Design review of the part built by this model. Coordinates are the model's own, in mm. Coordinates: 2 decimals unless noted, no trailing zeros. Loops run counter-clockwise (first coordinate to the right, second up) from the corner with the lowest first, then second, coordinate; pieces in that order, holes last. Notation, with made-up numbers: M -26,63 L -6,63 A20 ccw -6,87 Z; hole C 56.25,3 d10. An arc over 180 degrees is marked long. Write item = value, one per line. Start each with the question number.
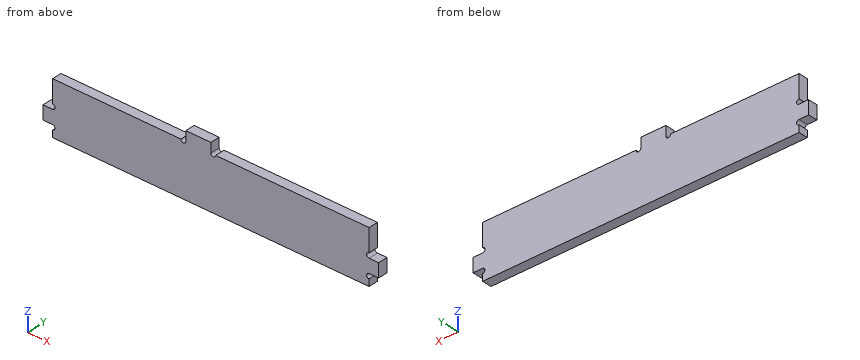
Autodesk Inventor part; units mm, degrees
ref_plane "YZ Plane" through (0, 0, 0) normal (1, 0, 0) x (0, 1, 0)
ref_plane "XZ Plane" through (0, 0, 0) normal (0, 1, 0) x (-1, 0, 0)
ref_plane "XY Plane" through (0, 0, 0) normal (0, 0, 1) x (1, 0, 0)
sketch "Sketch1" plane through (0, 0, 0) normal (0, 1, 0) x (-1, 0, 0)
  arc A0 (54.4292, -38.5976) -> (54.4292, -42.0976) centre (54.4292, -40.3476) ccw
  arc A1 (54.4292, -25.0976) -> (54.4292, -28.5976) centre (54.4292, -26.8476) ccw
  line L0 (61.4292, -38.5976) -> (61.4292, -28.5976)
  line L1 (-42.6541, -8.5976) -> (-42.6541, -1.5976)
  line L2 (61.4292, -28.5976) -> (54.4292, -28.5976)
  line L3 (61.4292, -38.5976) -> (54.4292, -38.5976)
  line L4 (54.4292, -25.0976) -> (54.4292, -8.5976)
  line L5 (54.4292, -42.0976) -> (54.4292, -47.0976)
  line L6 (-60.9041, -44.0976) -> (-60.9041, -33.5976)
  arc A2 (-176.2375, -42.0976) -> (-176.2375, -38.5976) centre (-176.2375, -40.3476) ccw
  arc A3 (-176.2375, -28.5976) -> (-176.2375, -25.0976) centre (-176.2375, -26.8476) ccw
  line L7 (-183.2375, -38.5976) -> (-183.2375, -28.5976)
  line L8 (-183.2375, -28.5976) -> (-176.2375, -28.5976)
  line L9 (-183.2375, -38.5976) -> (-176.2375, -38.5976)
  line L10 (-176.2375, -25.0976) -> (-176.2375, -8.5976)
  line L11 (-176.2375, -42.0976) -> (-176.2375, -47.0976)
  line L12 (54.4292, -47.0976) -> (-176.2375, -47.0976)
  arc A4 (-42.6541, -8.5976) -> (-39.1541, -8.5976) centre (-40.9041, -8.5976) ccw
  line L13 (-39.1541, -8.5976) -> (54.4292, -8.5976)
  line L14 (-60.9041, -1.5976) -> (-60.9041, -8.5976)
  arc A5 (-64.4041, -8.5976) -> (-60.9041, -8.5976) centre (-62.6541, -8.5976) ccw
  line L15 (-64.4041, -8.5976) -> (-176.2375, -8.5976)
  line L16 (-42.6541, -1.5976) -> (-60.9041, -1.5976)
  point P0 (0, 0)
  dimension "d2" = 3.5
  dimension "d5" = 3.5
  dimension "d9" = 7
  dimension "d11" = 10
  dimension "d32" = 5
  dimension "d33" = 230.6667
  dimension "d36" = 7
  dimension "d42" = 3.5
  dimension "d43" = 97.0833
  dimension "d44" = 3.5
  dimension "d45" = 18.25
  dimension "d46" = 20
extrude "Extrusion1" add sketch "Sketch1" along normal blind 7
properties part number "Level 1 Support Mid" material "Wood (Maple)"
(1) Take a section at A-A (y = 4.5). State the section outline as (x, z) points.
(2) Insertion check: pin 1 (1.5 mm diameter, centred on y = 2.5, z = -21.5, fed in from +X); pin 2 (2 mm diameter, centred on y = 2, z = -18.5, fed in from -X); pin 3 (2 mm diameter, centred on x = 181.5, y = 3.5, fed in from -Z). Each pin has a flat end and moves straight along its axis. Give the tip position at first contact, or say it passes through.
(3) To check wall thickness, follow L1, parallel to Z at x = 154, y = 5; L2, parallel to X at y = 3.75, z = -24; L3, parallel to X at y = 6.75, z = -4. State the ranges of each line that lie inside material, in increasing order.
(4) Take a section at B-B (x = 126.5). State the section outline as (y, z) points.
(5) Take a section at C-C (z = -15). State the section outline as (x, y) points, plus the area to 3 significant figures.
Results list:
q1.outline = M -61.43,-38.6 L -54.43,-38.6 A1.75 cw -54.43,-42.1 L -54.43,-47.1 L 176.24,-47.1 L 176.24,-42.1 A1.75 cw 176.24,-38.6 L 183.24,-38.6 L 183.24,-28.6 L 176.24,-28.6 A1.75 cw 176.24,-25.1 L 176.24,-8.6 L 64.4,-8.6 A1.75 cw 60.9,-8.6 L 60.9,-1.6 L 42.65,-1.6 L 42.65,-8.6 A1.75 cw 39.15,-8.6 L -54.43,-8.6 L -54.43,-25.1 A1.75 cw -54.43,-28.6 L -61.43,-28.6 Z
q2.pin_1 = 176.24
q2.pin_2 = -54.43
q2.pin_3 = -38.6
q3.L1 = -47.1 to -8.6
q3.L2 = -54.43 to 176.24
q3.L3 = 42.65 to 60.9
q4.outline = M 0,-47.1 L 7,-47.1 L 7,-8.6 L 0,-8.6 Z
q5.outline = M -54.43,0 L 176.24,0 L 176.24,7 L -54.43,7 Z
q5.area = 1,610 mm^2
